Here's how the part is built. I have some questions about the finished solid (model axes, mm). A direction names the side the tool comes from. Round coordinates to 2 decimals unless told otherwise and drop trailing zeros. Write each loop counter-clockwise with the first axis right and the second up, starting at its lowest first coordinate (ties: lowest second). Pieces come first, ordered by that corner, then holes. Notation, with made-up numbers: M 63.25,25.5 L 92.25,25.5 A14 ccw 92.25,42.5 Z; hole C 11.25,42 d11. An arc over 180 degrees is marked long. Use one line per item in the form item = value. Start each with the question number.
Q1. I'm going to push flat-ended pins straight in: pin 1 Ø3 at (y, z) = (80, 5) entering from -X; pin 2 Ø1.7 at (y, z) = (88.5, 4.5) entering from -X; pin 3 Ø4 at (x, z) = (-77.5, 3) entering from -Y. Where does each tip first touch, or does it pass through?
Q2. For faces 1 (the face through (-61, 62, 2)), 2 (the face through (-65.1, 67.14, 1.52)), 3 (the face through (-61, 68, 5)), which set-ups out of +Z, -Z, +X, -X, +Y, -Y let a thin tool reach every point of the face, with its end or its side?
Q3. We'd pull the mould along X, two halves only. Please class faces 4 (the face through (-62.6, 83.9, 8)), 5 (the face through (-60, 79, 4)), 6 (the face through (-85.8, 89, 4)): +X half, -X half, draft (parallel to the pull), parting line (faces both ways), or undercut.
Q4. I want a section at C-C on z = 7.25. List the corners of the cut face in (x, y) for me.
Q5. I want a section at B-B on x = -62.5. List the corners of the cut face in (y, z) for me.
Q6. I need wall thicknesses on line 1 along X through (y, z) = (65, 1.8); line 2 along X through (y, z) = (73.5, 6.25); line 3 along Y through (x, z) = (-74.5, 7.5). Which ranges of each line are inside material? Lowest first, please. Write a range as from..to.
Q7. I want a section at D-D on y = 72.75. List the corners of the cut face in (x, z) for me.
Q8. I want a section at A-A on y = 64.25. List the corners of the cut face in (x, z) for me, and give its area (3 significant figures).
Autodesk Inventor part; units mm, degrees
ref_plane "YZ Plane" through (0, 0, 0) normal (1, 0, 0) x (0, 1, 0)
ref_plane "XZ Plane" through (0, 0, 0) normal (0, 1, 0) x (-1, 0, 0)
ref_plane "XY Plane" through (0, 0, 0) normal (0, 0, 1) x (1, 0, 0)
sketch "Sketch1" plane through (0, 0, 0) normal (0, 0, 1) x (1, 0, 0)
  line L0 (-58, -60) -> (-60, -60)
  line L1 (-60, -60) -> (-60, -39.5)
  line L2 (-60, -39.5) -> (-58, -39.5)
  line L3 (-58, -39.5) -> (-58, -60)
  line L4 (49.6, 30) -> (51.6, 30)
  line L5 (51.6, 30) -> (51.6, 9.5)
  line L6 (51.6, 9.5) -> (49.6, 9.5)
  line L7 (49.6, 9.5) -> (49.6, 30)
  line L8 (-58, 39.5) -> (-60, 39.5)
  line L9 (-60, 39.5) -> (-60, 60)
  line L10 (-60, 60) -> (-58, 60)
  line L11 (-58, 60) -> (-58, 39.5)
  line L12 (-21.6, -39.5) -> (-19.6, -39.5)
  line L13 (-19.6, -39.5) -> (-19.6, -60)
  line L14 (-19.6, -60) -> (-21.6, -60)
  line L15 (-21.6, -60) -> (-21.6, -39.5)
  line L16 (51.6, -30) -> (49.6, -30)
  line L17 (49.6, -30) -> (49.6, -9.5)
  line L18 (49.6, -9.5) -> (51.6, -9.5)
  line L19 (51.6, -9.5) -> (51.6, -30)
  line L20 (-21.6, 60) -> (-19.6, 60)
  line L21 (-19.6, 60) -> (-19.6, 39.5)
  line L22 (-19.6, 39.5) -> (-21.6, 39.5)
  line L23 (-21.6, 39.5) -> (-21.6, 60)
  line L24 (90, -35) -> (90, 35)
  line L25 (90, 35) -> (49.6, 35)
  line L26 (49.6, 35) -> (49.6, 60)
  line L27 (49.6, 60) -> (90, 60)
  line L28 (90, 60) -> (90, 90)
  line L29 (90, 90) -> (-19.6, 90)
  line L30 (-19.6, 90) -> (-19.6, 65)
  line L31 (-19.6, 65) -> (-60, 65)
  line L32 (-60, 65) -> (-60, 90)
  line L33 (-60, 90) -> (-90, 90)
  line L34 (-90, 90) -> (-90, -90)
  line L35 (-90, -90) -> (-60, -90)
  line L36 (-60, -90) -> (-60, -65)
  line L37 (-60, -65) -> (-19.6, -65)
  line L38 (-19.6, -65) -> (-19.6, -90)
  line L39 (-19.6, -90) -> (90, -90)
  line L40 (90, -90) -> (90, -60)
  line L41 (90, -60) -> (49.6, -60)
  line L42 (49.6, -60) -> (49.6, -35)
  line L43 (49.6, -35) -> (90, -35)
  line L44 (86, -32) -> (73.8, -32)
  line L45 (73.8, -32) -> (73.8, -7.5)
  line L46 (73.8, -7.5) -> (86, -7.5)
  line L47 (86, -7.5) -> (86, -32)
  line L48 (65.8, -32) -> (53.6, -32)
  line L49 (53.6, -32) -> (53.6, -7.5)
  line L50 (53.6, -7.5) -> (65.8, -7.5)
  line L51 (65.8, -7.5) -> (65.8, -32)
  line L52 (86, -86) -> (70.6, -86)
  line L53 (70.6, -86) -> (70.6, -69.8)
  line L54 (70.6, -69.8) -> (86, -69.8)
  line L55 (86, -69.8) -> (86, -86)
  line L56 (86, 86) -> (86, 69.8)
  line L57 (86, 69.8) -> (70.6, 69.8)
  line L58 (70.6, 69.8) -> (70.6, 86)
  line L59 (70.6, 86) -> (86, 86)
  line L60 (73.8, 32) -> (86, 32)
  line L61 (86, 32) -> (86, 7.5)
  line L62 (86, 7.5) -> (73.8, 7.5)
  line L63 (73.8, 7.5) -> (73.8, 32)
  line L64 (65.8, 32) -> (65.8, 7.5)
  line L65 (65.8, 7.5) -> (53.6, 7.5)
  line L66 (53.6, 7.5) -> (53.6, 32)
  line L67 (53.6, 32) -> (65.8, 32)
  line L68 (-69.6, -87) -> (-85, -87)
  line L69 (-85, -87) -> (-85, -70.8)
  line L70 (-85, -70.8) -> (-69.6, -70.8)
  line L71 (-69.6, -70.8) -> (-69.6, -87)
  line L72 (-56, -62) -> (-56, -37.5)
  line L73 (-56, -37.5) -> (-43.8, -37.5)
  line L74 (-43.8, -37.5) -> (-43.8, -62)
  line L75 (-43.8, -62) -> (-56, -62)
  line L76 (-56, 62) -> (-43.8, 62)
  line L77 (-43.8, 62) -> (-43.8, 37.5)
  line L78 (-43.8, 37.5) -> (-56, 37.5)
  line L79 (-56, 37.5) -> (-56, 62)
  line L80 (-23.6, 62) -> (-23.6, 37.5)
  line L81 (-23.6, 37.5) -> (-35.8, 37.5)
  line L82 (-35.8, 37.5) -> (-35.8, 62)
  line L83 (-35.8, 62) -> (-23.6, 62)
  line L84 (-23.6, -62) -> (-35.8, -62)
  line L85 (-35.8, -62) -> (-35.8, -37.5)
  line L86 (-35.8, -37.5) -> (-23.6, -37.5)
  line L87 (-23.6, -37.5) -> (-23.6, -62)
  line L88 (-85, 87) -> (-69.6, 87)
  line L89 (-69.6, 87) -> (-69.6, 70.8)
  line L90 (-69.6, 70.8) -> (-85, 70.8)
  line L91 (-85, 70.8) -> (-85, 87)
  line L92 (-90, 90) -> (-60, 90)
  line L93 (-60, 90) -> (-60, 87)
  line L94 (-60, 87) -> (-90, 87)
  line L95 (-90, 87) -> (-90, 90)
  line L96 (-90, 90) -> (-60, 90)
  line L97 (-60, 90) -> (-60, 87)
  line L98 (-60, 87) -> (-90, 87)
  line L99 (-90, 87) -> (-90, 90)
  line L100 (-19.6, 65) -> (-60, 65)
  line L101 (-60, 65) -> (-60, 68)
  line L102 (-60, 68) -> (-63, 68)
  line L103 (-63, 62) -> (-16.6, 62)
  line L104 (-19.6, 68) -> (-19.6, 65)
  line L105 (-60, 87) -> (-63, 87)
  line L106 (-63, 87) -> (-63, 68)
  line L107 (-63, 68) -> (-60, 68)
  line L108 (-60, 68) -> (-60, 87)
  circle A0 centre (-63, -65) radius 1.5
  circle A1 centre (-16.6, -87) radius 1.5
  circle A2 centre (49.6, -87) radius 1.5
  circle A3 centre (46.6, -60) radius 1.5
  circle A4 centre (87, -63) radius 1.5
  circle A5 centre (46.6, -32) radius 1.5
  circle A6 centre (46.6, 32) radius 1.5
  circle A7 centre (87, 63) radius 1.5
  circle A8 centre (46.6, 60) radius 1.5
  circle A9 centre (49.6, 87) radius 1.5
  circle A10 centre (-16.6, 87) radius 1.5
  circle A11 centre (-16.6, 65) radius 1.5
  circle A12 centre (-63, 65) radius 1.5
  arc A13 (-63, 68) -> (-63, 62) centre (-63, 65) ccw
  arc A14 (-16.6, 62) -> (-16.6, 68) centre (-16.6, 65) ccw
  line L109 (-16.6, 68) -> (-19.6, 68)
  line L110 (-76, -39.25) -> (-82, -39.25)
  line L111 (-82, -39.25) -> (-82, -20.75)
  line L112 (-82, -20.75) -> (-76, -20.75)
  line L113 (-76, -20.75) -> (-76, -39.25)
  line L114 (-76, 20.75) -> (-82, 20.75)
  line L115 (-82, 20.75) -> (-82, 39.25)
  line L116 (-82, 39.25) -> (-76, 39.25)
  line L117 (-76, 39.25) -> (-76, 20.75)
  circle A15 centre (-87, 55.8) radius 1.25
  circle A16 centre (-87, -55.8) radius 1.25
  point P0 (0, 0)
extrude "Extrusion1" add sketch "Sketch1" along normal blind 8 contours L102 L106 L94 L32 | L34 L33 L32 L94 L88
sketch "Sketch2" plane through (-63, 68, 0) normal (-1, 0, 0) x (0, 0, 1)
  line L0 (0, 0) -> (3, 0)
  line L1 (3, 0) -> (3, -6)
  line L2 (3, -6) -> (0, -6)
  line L3 (0, -6) -> (0, 0)
  point P0 (0, -68)
  dimension "d2" = 3
  dimension "d3" = 6
extrude "Extrusion2" add sketch "Sketch2" along normal mid plane 6
sketch "Sketch3" plane through (-66, 62, 3) normal (0, 0, 1) x (1, 0, 0)
  circle A0 centre (3, 3) radius 2
  circle A1 centre (3, 3) radius 1.65
  point P0 (66, -62)
  dimension "d6" = 3.3
extrude "Extrusion3" cut sketch "Sketch3" against normal blind 3 contours A1
sketch "Sketch4" plane through (-90, 90, 0) normal (0, 1, 0) x (1, 0, 0)
  line L0 (0, 0) -> (27, 0)
  line L1 (0, 0) -> (0, -3.137)
  line L2 (0, 0) -> (0, -8)
  line L3 (0, -3.137) -> (9.9706, -8)
  line L4 (0, -3.137) -> (11.0933, -3.137) construction
  line L5 (30, -8) -> (0, -8)
  point P0 (90, 0)
  dimension "d9" = 3.137
  dimension "d10" = 26
extrude "Extrusion4" cut sketch "Sketch4" against normal blind 3
fillet "Fillet1" radius 3 2 edges at (-66, 62, 1.5) (-66, 68, 1.5)
sketch "Sketch5" plane through (-90, 90, 0) normal (0, 1, 0) x (1, 0, 0)
  circle A0 centre (3, -3.6) radius 1.2
  line L0 (4.2, -4.8) -> (1.8, -4.8)
  line L1 (1.8, -4.8) -> (1.8, -2.4)
  line L2 (1.8, -2.4) -> (4.2, -2.4)
  line L3 (4.2, -2.4) -> (4.2, -4.8)
  line L4 (4.2, -4.8) -> (1.8, -2.4) construction
  line L5 (1.8, -4.8) -> (4.2, -2.4) construction
  line L6 (4.2, -4.8) -> (4.2, -5.1855)
  line L7 (9.9706, -8) -> (0, -3.137)
  line L8 (4.2, -5.1855) -> (3.3204, -4.7564)
  point P0 (90, 0)
  point P1 (4.2, -3.6)
  point P2 (3, -2.4)
  point P3 (3, -4.8)
  point P4 (1.8, -3.6)
  point P5 (3.4097, -4.8)
  point P6 (1.8, -4.0149)
extrude "Extrusion5" cut sketch "Sketch5" against normal blind 3 contours L7 A0 | A0 L3 L0 L7 | L0 L6 L7 | L7 L1 A0 picked at (3.1852, -3.7592)
properties part number "leftfrontwall"
Reported:
q1.pin_1 = -63
q1.pin_2 = -88.95
q1.pin_3 = 87
q2.face_1 = +Z, -Z, +X, -X, -Y
q2.face_2 = +Z, -Z, -X
q2.face_3 = +Z, +X, -X, -Y
q3.face_4 = draft
q3.face_5 = +X half
q3.face_6 = undercut
q4.outline = M -81.57,87 L -63,87 L -63,68 L -60,68 L -60,90 L -81.57,90 Z
q5.outline = M 62,0 L 63.43,0 L 63.43,3 L 62,3 Z; M 66.57,0 L 90,0 L 90,8 L 68,8 L 68,3 L 66.57,3 Z
q6.line_1 = -66..-64.65, -61.35..-60
q6.line_2 = -63..-60
q6.line_3 = 87..90
q7.outline = M -63,0 L -60,0 L -60,8 L -63,8 Z
q8.outline = M -65.9,0 L -64.47,0 L -64.47,3 L -65.9,3 Z; M -61.53,0 L -60,0 L -60,3 L -61.53,3 Z
q8.area = 8.90 mm^2
